```python
from build123d import *

# Parameters (mm, degrees)
SALIENTE_EXTRUIR1_DEPTH = 100
CROQUIS3_W              = 10
CROQUIS3_H              = 6
SALIENTE_EXTRUIR2_DEPTH = 1.2
CROQUIS4_W              = 10
CROQUIS4_H              = 6
SALIENTE_EXTRUIR3_DEPTH = 1.2
CROQUIS5_R              = 1.5
CORTAR_EXTRUIR1_DEPTH   = 119.841982146
CROQUIS6_W              = 18
CROQUIS6_H              = 10.2
CORTAR_EXTRUIR2_DEPTH   = 14


with BuildPart() as part:
    # Croquis1 → Saliente-Extruir1 (new body)
    with BuildSketch(Plane(origin=(0, 0, 0), x_dir=(0, 0, -1), z_dir=(1, 0, 0))):
        Polygon((0, 0), (1.2, 0), (15.512007455, 58.268056795), (14.312007455, 58.268056795), align=None)
    extrude(amount=-SALIENTE_EXTRUIR1_DEPTH)

    # Croquis3 → Saliente-Extruir2 (add)
    with BuildSketch(Plane(origin=(0, 0, 0), x_dir=(0, 0, -1), z_dir=(1, 0, 0))):
        with Locations((10.572099341, 20.8)):
            Rectangle(CROQUIS3_W, CROQUIS3_H)
    extrude(amount=SALIENTE_EXTRUIR2_DEPTH)

    # Croquis4 → Saliente-Extruir3 (add)
    with BuildSketch(Plane.ZY.offset(100)):
        with Locations((-10.572099341, 20.8)):
            Rectangle(CROQUIS4_W, CROQUIS4_H)
    extrude(amount=SALIENTE_EXTRUIR3_DEPTH)

    # Croquis5 → Cortar-Extruir1 (cut, through all)
    with BuildSketch(Plane(origin=(1.2, 0, 0), x_dir=(0, 0, -1), z_dir=(1, 0, 0))):
        with Locations((10.308970016, 20.8)):
            Circle(CROQUIS5_R)
    extrude(amount=-CORTAR_EXTRUIR1_DEPTH, mode=Mode.SUBTRACT)

    # Croquis6 → Cortar-Extruir2 (cut)
    with BuildSketch(Plane(origin=(0, 0, 0), x_dir=(1, 0, 0), z_dir=(0, 0.2385334575785815, 0.971134279909636))):
        with Locations((-81, 17.1)):
            Rectangle(CROQUIS6_W, CROQUIS6_H)
        with Locations((-19, 17.1)):
            Rectangle(CROQUIS6_W, CROQUIS6_H)
    extrude(amount=-CORTAR_EXTRUIR2_DEPTH, mode=Mode.SUBTRACT)


solid = part.part
```
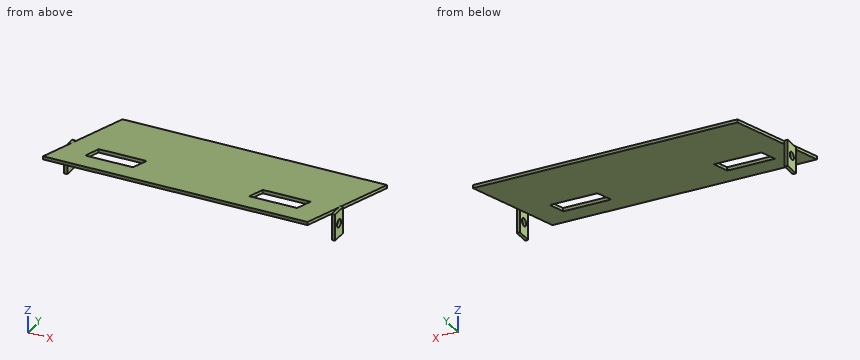
CAD build for the part. Positions are in the model's coordinates, mm. Coordinates: 2 decimals unless noted, no trailing zeros. Write each loop counter-clockwise with the first axis right and the second up, starting at its lowest first coordinate (ties: lowest second). Pieces come first, ordered by that corner, then holes. Notation, with made-up numbers: (50, -25) -> (73, -25) arc R12 cw to (73, -2) -> close; hole circle Ø9 at (87, 46.5). An arc over 180 degrees is marked (long way). Return JSON: item names as keys, results as strings. Group by question number.
Q1. Cut at B-B, the plane x = -55.5. Give the cut face in (y, z).
Q2. Cut at A-A, the plane x = -15. Give the cut face in (y, z), then the cut area to 3 significant figures.
Q3. Flat gauge pins, fed straight in: pin 1 (1 mm diameter, centred on x = -101, z = -11, fed in from +Y); pin 2 (4 mm diameter, centred on x = -75.5, y = 36, fed in from -Z); pin 3 (1 mm diameter, centred on x = 1, z = -10.5, fed in from -Y). Where does each tip first touch, or does it go through?
Q4. Cut at C-C, the plane y = 46. Give the cut face in (x, z), then the cut area to 3 significant figures.
Q5. Drill centre lines: line 1 (X direction, y = 20.5, z = -12.5); line 2 (X direction, y = 50, z = -12.75); line 3 (Z direction, x = -30.5, y = 36). Where is each one in solid material? Low to high.
Returned:
{
 "1": {"outline": "(0, -1.2) -> (58.27, -15.51) -> (58.27, -14.31) -> (0, 0) -> close"},
 "2": {"outline": "(0, -1.2) -> (11.38, -3.99) -> (11.65, -2.86) -> (0, 0) -> close; (21.28, -6.43) -> (58.27, -15.51) -> (58.27, -14.31) -> (21.56, -5.3) -> close", "area": "58.0 mm2"},
 "3": {"pin 1": "stops at y = 23.8", "pin 2": "stops at z = -10.53", "pin 3": "stops at y = 17.8"},
 "4": {"outline": "(-100, -12.5) -> (0, -12.5) -> (0, -11.3) -> (-100, -11.3) -> close", "area": "120 mm2"},
 "5": {"line 1": "x = -101.2 to -100, 0 to 1.2", "line 2": "x = -100 to 0", "line 3": "z = -10.04 to -8.84"}
}
